Autodesk Inventor part; units mm, degrees
ref_plane "YZ Plane" through (0, 0, 0) normal (1, 0, 0) x (0, 1, 0)
ref_plane "XZ Plane" through (0, 0, 0) normal (0, 1, 0) x (-1, 0, 0)
ref_plane "XY Plane" through (0, 0, 0) normal (0, 0, 1) x (1, 0, 0)
sketch "Skizze1" plane through (0, 0, 0) normal (0, 0, 1) x (1, 0, 0)
  circle A0 centre (0, 0) radius 8
  line L0 (0, -8) -> (0, 8)
  dimension "d0" = 16
extrude "Extrusion1" add sketch "Skizze1" along normal blind 14 contours L0 A0 picked at (-4.0721, -1.7428)
sketch "Skizze2" plane through (0, -8, 0) normal (1, 0, 0) x (0, 0, -1)
  line L0 (0, 0) -> (0, 16) construction
  line L1 (0, 16) -> (-14, 16) construction
  line L2 (-14, 0) -> (-14, 16) construction
  line L3 (0, 0) -> (-14, 0) construction
  line L4 (-14, 16) -> (-14, 0) construction
  line L5 (0, 16) -> (0, 0) construction
  line L6 (-14, 16) -> (0, 0) construction
  line L7 (0, 0) -> (-14, 0) construction
  line L8 (-14, 0) -> (0, 16) construction
  line L9 (-14, 8) -> (0, 8) construction
  point P0 (-4, 8)
  dimension "d12" = 4
hole "Bohrung1" at (0, 0, 4) direction (-1, 0, 0) diameter 5.5 end through all
sketch "Skizze3" plane through (0, -8, 0) normal (1, 0, 0) x (0, 0, -1)
  circle A0 centre (-4, 8) radius 2.75
  line L0 (-4, 5.25) -> (0, 5.25)
  line L1 (0, 16) -> (0, 0) construction
  line L2 (-4, 10.75) -> (0, 10.75)
  line L3 (0, 5.25) -> (0, 10.75)
  circle A1 centre (-4, 8) radius 2.75 construction
  point P0 (0, 8)
extrude "Extrusion2" cut sketch "Skizze3" against normal through all contours A0 L2 L3 L0
properties part number "Gabel_Enforcement"
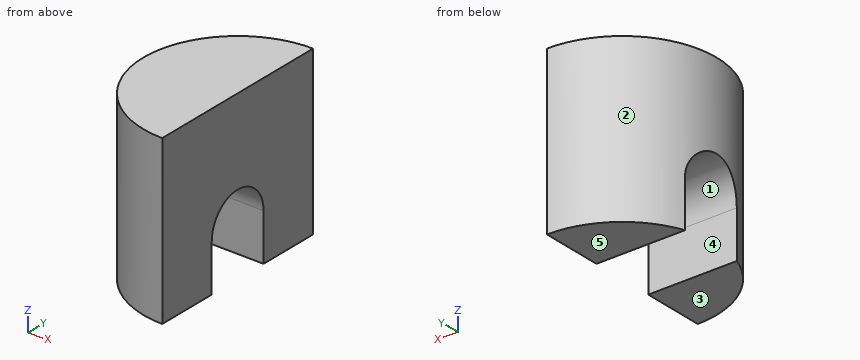
Could you check a few things on this model? Use its own coordinates, in mm. Face numbers are marked on the shaded views. A direction names the side the tool comes from. Round coordinates to 2 decimals unless told otherwise and drop trailing zeros. Order: outer loops, then holes, each group sorted by start corner. A loop starts at its lowest first (then second) coordinate and runs counter-clockwise, first axis right, second up.
(1) If we mould it in two halves opening along Y, with no side actions, what happens to the marked faces 1, 2 and 3? For each: released by +Y, released by -Y, zero draft, split by the parting line, or undercut.
Response values:
face 1: undercut
face 2: split by the parting line
face 3: zero draft
(2) Imagine slicing it at B-B (x = -0.5). Write out the boundary of the cut face in (y, z), plus the area to 3 significant figures.
Response values:
outline: (-7.98, 0) - (-2.75, 0) - (-2.75, 4) arc R2.75 cw to (2.75, 4) - (2.75, 0) - (7.98, 0) - (7.98, 14) - (-7.98, 14) - close
area: 190 mm2
(3) Imagine slicing it at C-C (y = 0). Write out the boundary of the cut face in (x, z).
Response values:
outline: (-8, 6.75) - (0, 6.75) - (0, 14) - (-8, 14) - close
(4) Please list where these lines run through material, in increasing order: line 1 along Y through (x, z) = (-2.5, 5); line 2 along Y through (x, z) = (-1, 5.75); line 3 along X through (y, z) = (7, 1.5).
Response values:
line 1: y = -7.6 to -2.56, 2.56 to 7.6
line 2: y = -7.94 to -2.12, 2.12 to 7.94
line 3: x = -3.87 to 0
(5) Imagine slicing it at D-D (z = 12.25). Write out the boundary of the cut face in (x, y), plus the area to 3 significant figures.
Response values:
outline: (0, -8) - (0, 8) arc R8 ccw to start
area: 101 mm2
(6) Imagine slicing it at A-A (z = 1.25). Write out the boundary of the cut face in (x, y), plus the area to 3 significant figures.
Response values:
outline: (-7.51, -2.75) arc R8 ccw to (0, -8) - (0, -2.75) - close; (-7.51, 2.75) - (0, 2.75) - (0, 8) arc R8 ccw to start
area: 57.4 mm2
(7) I'm going to push flat-ended pins straight in: pin 1 (4.5 mm diameter, centred on x = -5, z = 2.5, fed in from +Y); pin 2 (4.5 mm diameter, centred on x = -4, z = 2, fed in from -Y); pin 3 (1.5 mm diameter, centred on x = -7, z = 5, fed in from +Y). Where does each tip first touch, or does it pass through?
Response values:
pin 1: stops at y = 7.51
pin 2: stops at y = -7.81
pin 3: stops at y = 4.99
(8) Which directions (+Z, -Z, +X, -X, +Y, -Y) give clear straight access to the entire face, cutting with the end or side of a thin tool? Please do the marked faces 4 and 5.
Response values:
face 4: -Z, +X, -X
face 5: -Z, +X, -X, +Y, -Y
